from build123d import *

# Parameters (mm, degrees)
SKETCH1_W           = 55
SKETCH1_H           = 60
BOSS_EXTRUDE1_DEPTH = 40
SKETCH2_R           = 4
BOSS_EXTRUDE2_DEPTH = 7
SKETCH4_W           = 40
SKETCH4_H           = 25
BOSS_EXTRUDE3_DEPTH = 25
SKETCH5_R           = 5
BOSS_EXTRUDE4_DEPTH = 35
BOSS_EXTRUDE5_DEPTH = 10


with BuildPart() as part:
    # Sketch1 → Boss-Extrude1 (new body)
    with BuildSketch(Plane.XY):
        Rectangle(SKETCH1_W, SKETCH1_H)
    extrude(amount=BOSS_EXTRUDE1_DEPTH)

    # Sketch2 → Boss-Extrude2 (add)
    with BuildSketch(Plane(origin=(0, 30, 0), x_dir=(-1, 0, 0), z_dir=(0, 1, 0))):
        with Locations((0, 20)):
            Circle(SKETCH2_R)
    extrude(amount=BOSS_EXTRUDE2_DEPTH)

    # Sketch4 → Boss-Extrude3 (add)
    with BuildSketch(Plane(origin=(0, 37, 0), x_dir=(1, 0, 0), z_dir=(0, 1, 0))):
        with Locations((0, -20)):
            Rectangle(SKETCH4_W, SKETCH4_H)
    extrude(amount=BOSS_EXTRUDE3_DEPTH)

    # Sketch5 → Boss-Extrude4 (add)
    with BuildSketch(Plane.XZ.offset(30)):
        with Locations((-14, 20)):
            Circle(SKETCH5_R)
        with Locations((14, 20)):
            Circle(SKETCH5_R)
    extrude(amount=BOSS_EXTRUDE4_DEPTH)

    # Sketch6 → Boss-Extrude5 (add)
    with BuildSketch(Plane.XZ.offset(65)):
        Polygon((-11.888014897, 12.878679656), (-6.888014897, 17.878679656), (-4.829546686, 19.937147868), (-6.888014897, 22.121320344), (-11.888014897, 27.121320344), (-16.837762365, 32.071067812), (-18.959082709, 29.949747468), (-23.959082709, 24.949747468), (-26.080403052, 22.828427125), (-21.130655584, 17.878679656), (-16.130655584, 12.878679656), (-14.009335241, 10.757359313), align=None)
        Polygon((18.949747468, 29.949747468), (23.949747468, 24.949747468), (26.071067812, 22.828427125), (21.121320344, 17.878679656), (16.121320344, 12.878679656), (14, 10.757359313), (11.878679656, 12.878679656), (6.878679656, 17.878679656), (4.820211445, 19.937147868), (6.878679656, 22.121320344), (11.878679656, 27.121320344), (16.828427125, 32.071067812), align=None)
    extrude(amount=BOSS_EXTRUDE5_DEPTH)


solid = part.part
CAD build for the part. Positions are in the model's coordinates, mm. A direction names the side the tool comes from. Give positions to 0.01 mm unless a question says otherwise; leave off trailing zeros. Loops run counter-clockwise (first coordinate to the right, second up) from the corner with the lowest first, then second, coordinate; pieces in that order, holes last. Notation, with made-up numbers: M 76,34 L 108,34 A11 ccw 108,41 Z; hole C 67.25,45 d1. An arc over 180 degrees is marked long. One line per question, with ' | ' between items. Start each with the question number.
1. Saw through at D-D on z = 35. Give the cut face in (x, y), plus the area to 3 significant figures.
2. 3-axis set-ups, long thin cutter, end or side, ignore diameter. For faces 4 (the face through (0, 49, 7.5)), 5 (the face through (-21.394, -69.93, 27.514)), 6 (the face through (-11.793, -69.93, 27.027)), 7 (the face through (-19, -65, 22)): which of +Z, -Z, +X, -X, +Y, -Y reach the whole face in a straight line?
3. Saw through at A-A on x = 22.5. Give the cut face in (y, z), plus the area to 3 significant figures.
4. Two-plate mould, pull along X, no slides. Class faces 1 (the face through (16.307, -47.255, 15.564)), 2 (the face through (-20, 49, 20)), 3 (the face through (20, 49, 20)): pulls with the +X half, pulls with the -X half, needs draft (parallel to the pull), parting line crosses it, or undercut.
5. Flat gauge pins, fed straight in: pin 1 (2 mm diameter, centred on x = 5, z = 21.5, fed in from -Y); pin 2 (8 mm diameter, centred on x = 16.5, y = 47.5, fed in from +Z); pin 3 (7.5 mm diameter, centred on y = 53.5, z = 17.5, fed in from -X); pin 4 (1.5 mm diameter, centred on x = 3, z = 26.5, fed in from -Y). Where does each tip first touch, or does it go through?
6. Probe L1, parallel to Y at x = -11, z = 15; L2, parallel to Y at x = 20.5, z = 23.5; L3, parallel to Y at x = -8.5, z = 27. List the from-to ranges inside material, lowest first. Write a range as from..to.
7. Saw through at C-C on y = 39.5. Give the cut face in (x, z), plus the area to 3 significant figures.
8. Saw through at B-B on x = 0. Give the cut face in (y, z), plus the area to 3 significant figures.
Result sheet:
1) outline: M -27.5,-30 L 27.5,-30 L 27.5,30 L -27.5,30 Z | area: 3,300 mm^2
2) face 4: -Z, +X, -X, +Y | face 5: +Z, -X, -Y | face 6: +Z, -Y | face 7: none
3) outline: M -75,19.26 L -65,19.26 L -65,26.4 L -75,26.4 Z; M -30,0 L 30,0 L 30,40 L -30,40 Z | area: 2,470 mm^2
4) face 1: undercut | face 2: pulls with the -X half | face 3: pulls with the +X half
5) pin 1: stops at y = -75 | pin 2: stops at z = 32.5 | pin 3: stops at x = -20 | pin 4: stops at y = -30
6) L1: y = -75..-65, -30..30, 37..62 | L2: y = -75..-65, -30..30 | L3: y = -30..30, 37..62
7) outline: M -20,7.5 L 20,7.5 L 20,32.5 L -20,32.5 Z | area: 1,000 mm^2
8) outline: M -30,0 L 30,0 L 30,16 L 37,16 L 37,7.5 L 62,7.5 L 62,32.5 L 37,32.5 L 37,24 L 30,24 L 30,40 L -30,40 Z | area: 3,080 mm^2
